Design review of the part built by this model. Coordinates are the model's own, in mm. A direction names the side the tool comes from. Coordinates: 2 decimals unless noted, no trailing zeros. Write each loop counter-clockwise with the first axis right and the second up, starting at its lowest first coordinate (ties: lowest second). Pieces come first, ordered by that corner, then holes. Notation, with made-up numbers: (6.25, 7.25) - (29.25, 7.25) arc R8 ccw to (29.25, 15.25) - close; hole circle Ø3 at (85.25, -2.5). An arc over 180 degrees is marked (long way). Answer as a JSON object with one key per item and string values.
```python
from build123d import *

# Parameters (mm, degrees)
SKETCH_1_R                          = 23
EXTRUDE_1_DEPTH                     = 4
CUT_EXTRUDE_1_DEPTH                 = 33.771939216
CUT_EXTRUDE_1_DEPTH_BACK            = 33.771939216
SKETCH_4_R                          = 16.25
CUT_EXTRUDE_2_DEPTH                 = 33.771939216
EXTRUDE_2_DEPTH                     = 3.5
FILLET_1_R                          = 5
EXTRUDE_START                       = -3.5
EXTRUDE_3_DEPTH                     = 27
CUT_EXTRUDE_START                   = -10
CUT_EXTRUDE_1_2_DEPTH               = 13.5
CHAMFER_1_SIZE                      = 0.5
HOLE_WIZARD_2_D                     = 4.5
HOLE_WIZARD_2_DEPTH                 = 7.5
HOLE_WIZARD_2_CBORE_D               = 7.5
HOLE_WIZARD_2_CBORE_DEPTH           = 3
HOLE_WIZARD_2_ON_FACE_2_D           = 4.5
HOLE_WIZARD_2_ON_FACE_2_DEPTH       = 7.5
HOLE_WIZARD_2_ON_FACE_2_CBORE_D     = 7.5
HOLE_WIZARD_2_ON_FACE_2_CBORE_DEPTH = 3
SKETCH_12_W                         = 0.1
SKETCH_12_H                         = 3
CUT_EXTRUDE_2_2_DEPTH               = 0.2


with BuildPart() as part:
    # 草图1 → 凸台-拉伸1 (new body)
    with BuildSketch(Plane(origin=(0, 0, 0), x_dir=(1, 0, 0), z_dir=(0, 1, 0))):
        with Locations(Location((0, 0, 0), (0, 0, 270))):
            Circle(SKETCH_1_R)
    extrude(amount=EXTRUDE_1_DEPTH)

    # 草图3 → Cut-Extrude 1 (cut, two sides: drawn at the far end of the back side and taken through both)
    with BuildSketch(Plane(origin=(0, 4, 0), x_dir=(1, 0, 0), z_dir=(0, 1, 0)).offset(-CUT_EXTRUDE_1_DEPTH_BACK)):
        Polygon((-121.379376924, 22.5), (-4.769696007, 22.5), (4.769696007, 22.5), (121.379376924, 22.5), (121.379376924, 255.719361835), (-121.379376924, 255.719361835), align=None)
    extrude(amount=CUT_EXTRUDE_1_DEPTH + CUT_EXTRUDE_1_DEPTH_BACK, mode=Mode.SUBTRACT)

    # 草图4 → Cut-Extrude 2 (cut, through all)
    with BuildSketch(Plane(origin=(0, 4, 0), x_dir=(1, 0, 0), z_dir=(0, 1, 0))):
        with Locations(Location((0, 0, 0), (0, 0, 270))):
            Circle(SKETCH_4_R)
    extrude(amount=-CUT_EXTRUDE_2_DEPTH, mode=Mode.SUBTRACT)

    # 草图5 → 凸台-拉伸2 (add)
    with BuildSketch(Plane(origin=(0, 0, 0), x_dir=(1, 0, 0), z_dir=(0, 1, 0))):
        with BuildLine():
            ThreePointArc((11.5, -19.918584287), (0, -23), (-11.5, -19.918584287))
            Line((-11.5, -19.918584287), (-17, -29.444863729))
            ThreePointArc((-17, -29.444863729), (0, -34), (17, -29.444863729))
            Line((17, -29.444863729), (11.5, -19.918584287))
        make_face()
    extrude(amount=EXTRUDE_2_DEPTH)

    # 圆角1
    fillet_1_edges = [part.edges().sort_by_distance(p)[0] for p in [
        (11.5, 1.75, 19.918584287),
        (-11.5, 1.75, 19.918584287),
    ]]
    fillet(fillet_1_edges, radius=FILLET_1_R)

    # 草图7 → 凸台-拉伸3 (add)
    with BuildSketch(Plane(origin=(0, 3.5, 0), x_dir=(1, 0, 0), z_dir=(0, 1, 0)).offset(EXTRUDE_START)):
        with BuildLine():
            Line((-14.5, -25.11473671), (-17, -29.444863729))
            ThreePointArc((-17, -29.444863729), (0, -34), (17, -29.444863729))
            Line((17, -29.444863729), (14.5, -25.11473671))
            ThreePointArc((14.5, -25.11473671), (0, -29), (-14.5, -25.11473671))
        make_face()
    extrude(amount=EXTRUDE_3_DEPTH)

    # 草图8 → Cut-Extrude 1 2 (cut)
    with BuildSketch(Plane(origin=(0, 27, 0), x_dir=(1, 0, 0), z_dir=(0, 1, 0)).offset(CUT_EXTRUDE_START)):
        with BuildLine():
            ThreePointArc((-14.75, -25.547749412), (0, -29.5), (14.75, -25.547749412))
            Line((14.75, -25.547749412), (14.25, -24.681724008))
            ThreePointArc((14.25, -24.681724008), (0, -28.5), (-14.25, -24.681724008))
            Line((-14.25, -24.681724008), (-14.75, -25.547749412))
        make_face()
    extrude(amount=-CUT_EXTRUDE_1_2_DEPTH, mode=Mode.SUBTRACT)

    # 倒角1
    chamfer_1_edges = [part.edges().sort_by_distance(p)[0] for p in [
        (0, 17, 29),
        (0, 27, 29),
    ]]
    chamfer(chamfer_1_edges, length=CHAMFER_1_SIZE - 0.0001)  # a hair under: the kernel refuses the full size

    # 孔2
    with Locations(Plane(origin=(8.799847533, 22, 32.841478094), x_dir=(0.965925826289, 0, -0.258819045103), z_dir=(0.258819045103, 0, 0.965925826289))):
        with Locations((1e-09, 0)):
            CounterBoreHole(HOLE_WIZARD_2_D / 2, HOLE_WIZARD_2_CBORE_D / 2, HOLE_WIZARD_2_CBORE_DEPTH, depth=HOLE_WIZARD_2_DEPTH)

    # 孔2 on face 2
    with Locations(Plane(origin=(-8.799847533, 22, 32.841478094), x_dir=(0.965925849201, 0, 0.258818959594), z_dir=(-0.258818959594, 0, 0.965925849201))):
        with Locations((-1e-09, 0)):
            CounterBoreHole(HOLE_WIZARD_2_ON_FACE_2_D / 2, HOLE_WIZARD_2_ON_FACE_2_CBORE_D / 2, HOLE_WIZARD_2_ON_FACE_2_CBORE_DEPTH, depth=HOLE_WIZARD_2_ON_FACE_2_DEPTH)

    # 草图12 → Cut-Extrude 2 2 (cut)
    with BuildSketch(Plane(origin=(0, 0, -22.5), x_dir=(-1, 0, 0), z_dir=(0, 0, -1))):
        with Locations((0, 2.5)):
            Rectangle(SKETCH_12_W, SKETCH_12_H)
    extrude(amount=-CUT_EXTRUDE_2_2_DEPTH, mode=Mode.SUBTRACT)


solid = part.part
```
(1) Take a section at B-B, the plane y = 12.5. Write out the cut boundary in (x, z), and give its area (3 significant figures).
Solved:
{"outline": "(-17, 29.44) - (-14.75, 25.55) arc R29.5 cw to (14.75, 25.55) - (17, 29.44) arc R34 ccw to start", "area": "150 mm^2"}
(2) Tool access review of faces 4 (the face through (-5.659, 22.053, 30.577)), 5 (the face through (0, 22, 29)), 6 (the face through (0, 27, 31)): name each direction out of +Z, -Z, +X, -X, +Y, -Y from which nothing blocks a thin tool from reaching the whole face with its end or side.
Solved:
{"face 4": "none", "face 5": "-Z, +Y", "face 6": "+Z, -Z, +X, -X, +Y"}
(3) The part is to be moulded in two halves that separate along Z. For faces 1 (the face through (0, 0, 18)), 2 (the face through (8.2, 19.8, 28.8)), 3 (the face through (-12.036, 22.165, 30.444)), say which applies: pulls with the +Z half, pulls with the -Z half, needs draft (parallel to the pull), parting line crosses it, or undercut.
Solved:
{"face 1": "needs draft", "face 2": "parting line crosses it", "face 3": "undercut"}
(4) Take a section at C-C, the plane x = 18. Write out the cut boundary in (y, z).
Solved:
{"outline": "(0, -14.32) - (4, -14.32) - (4, 14.32) - (0, 14.32) - close"}
(5) To check wall thickness, follow line 1 (X direction, y = 2.3, z = 0); line 2 (Y direction, x = -8.5, z = 26); line 3 (Y direction, x = 8, z = 30.5). State the ranges of each line that lie inside material, in increasing order. Write a range as from..to.
Solved:
{"line 1": "x = -23..-16.25, 16.25..23", "line 2": "y = 0..3.5", "line 3": "y = 0..18.25, 25.75..27"}
(6) Take a section at A-A, the plane z = 0. Write out the cut boundary in (x, y).
Solved:
{"outline": "(-23, 0) - (-16.25, 0) - (-16.25, 4) - (-23, 4) - close; (16.25, 0) - (23, 0) - (23, 4) - (16.25, 4) - close"}
(7) For pin 1 (1 mm diameter, centred on x = 16.5, z = -3.5, fed in from +Y); pin 2 (10 mm diameter, centred on y = 13.5, z = -11.5, fed in from -X); pin 3 (4 mm diameter, centred on x = -5.5, y = 17, fed in from +Z); pin 4 (4 mm diameter, centred on x = -11.5, y = 2.5, fed in from -Z), all flat-tipped, find the tip position at first contact; note any pin that passes through.
Solved:
{"pin 1": "stops at y = 4", "pin 2": "passes through", "pin 3": "stops at z = 33.82", "pin 4": "stops at z = -20.95"}
